from build123d import *

# Parameters (mm, degrees)
SKETCH1_R           = 11
BOSS_EXTRUDE1_DEPTH = 17.9
BOSS_EXTRUDE2_START = 32.2
SKETCH2_R           = 11
BOSS_EXTRUDE2_DEPTH = 32.2
BOSS_EXTRUDE3_DEPTH = 2.5
BOSS_EXTRUDE4_DEPTH = 15.3


# Read off the part's stored shape, not the designer's step: AdvancedHole1
with BuildPart() as part:
    # Sketch1 → Boss-Extrude1 (new body)
    with BuildSketch(Plane(origin=(0, 0, 0), x_dir=(0, 0, -1), z_dir=(1, 0, 0))):
        with Locations(Location((0, 0, 0), (0, 0, 180))):
            Circle(SKETCH1_R)
    extrude(amount=BOSS_EXTRUDE1_DEPTH)

    # Sketch2 → Boss-Extrude2 (add)
    with BuildSketch(Plane.ZY.offset(BOSS_EXTRUDE2_START)):
        Circle(SKETCH2_R)
    extrude(amount=-BOSS_EXTRUDE2_DEPTH)

    # Sketch3 → Cut-Revolve1 (revolve, cut)
    with BuildSketch(Plane.XY, mode=Mode.PRIVATE) as cut_revolve1_sk:
        with BuildLine():
            Line((0, 11), (0, 10))
            ThreePointArc((0, 10), (-0.292893219, 10.707106781), (-1, 11))
            Line((-1, 11), (0, 11))
        make_face()
    revolve(cut_revolve1_sk.sketch.rotate(Axis((17.9, 0, 0), (-1, 0, 0)), 270), axis=Axis((17.9, 0, 0), (-1, 0, 0)), mode=Mode.SUBTRACT)

    # Sketch4 → Boss-Extrude3 (add)
    with BuildSketch(Plane(origin=(17.9, 0, 0), x_dir=(0, 0, -1), z_dir=(1, 0, 0))):
        with BuildLine():
            ThreePointArc((4, 3), (2.236067977, 4.472135955), (0, 5))
            Line((0, 5), (0, -5))
            ThreePointArc((0, -5), (2.236067977, -4.472135955), (4, -3))
            Line((4, -3), (4, 3))
        make_face()
        with BuildLine():
            ThreePointArc((0, 5), (-2.236067977, 4.472135955), (-4, 3))
            Line((-4, 3), (-4, -3))
            ThreePointArc((-4, -3), (-2.236067977, -4.472135955), (0, -5))
            Line((0, -5), (0, 5))
        make_face()
    extrude(amount=BOSS_EXTRUDE3_DEPTH)

    # Sketch5 → Boss-Extrude4 (add)
    with BuildSketch(Plane(origin=(20.4, 0, 0), x_dir=(0, 0, -1), z_dir=(1, 0, 0))):
        with BuildLine():
            Line((0.968245837, 1.75), (-0.968245837, 1.75))
            ThreePointArc((-0.968245837, 1.75), (-1.015753003, -1.722859784), (2, 0))
            ThreePointArc((2, 0), (1.722859784, 1.015753003), (0.968245837, 1.75))
        make_face()
    extrude(amount=BOSS_EXTRUDE4_DEPTH)

    # AdvancedHole1 outline → AdvancedHole1 (revolve, cut)
    with BuildSketch(Plane(origin=(0, -9, 0), x_dir=(0, 1, 0), z_dir=(0, 0, -1))):
        Polygon((0, 14.219311505), (0.8, 14.7), (0.8, 17.9), (0, 17.9), align=None)
    revolve(axis=Axis((0, -9, 0), (1, 0, 0)), mode=Mode.SUBTRACT)

    # AdvancedHole1 2 outline → AdvancedHole1 2 (revolve, cut)
    with BuildSketch(Plane.YX.offset(9)):
        Polygon((0, 14.219311505), (0.8, 14.7), (0.8, 17.9), (0, 17.9), align=None)
    revolve(axis=Axis((0, 0, -9), (1, 0, 0)), mode=Mode.SUBTRACT)

    # AdvancedHole1 3 outline → AdvancedHole1 3 (revolve, cut)
    with BuildSketch(Plane.YX.offset(-9)):
        Polygon((0, 14.219311505), (0.8, 14.7), (0.8, 17.9), (0, 17.9), align=None)
    revolve(axis=Axis((0, 0, 9), (1, 0, 0)), mode=Mode.SUBTRACT)

    # AdvancedHole1 4 outline → AdvancedHole1 4 (revolve, cut)
    with BuildSketch(Plane(origin=(0, 9, 0), x_dir=(0, 1, 0), z_dir=(0, 0, -1))):
        Polygon((0, 14.219311505), (0.8, 14.7), (0.8, 17.9), (0, 17.9), align=None)
    revolve(axis=Axis((0, 9, 0), (1, 0, 0)), mode=Mode.SUBTRACT)


solid = part.part
Input: part model. Units: mm. Frame: model coordinates. A direction names the side the tool comes from. Coordinates: 2 decimals unless noted, no trailing zeros. Loops run counter-clockwise (first coordinate to the right, second up) from the corner with the lowest first, then second, coordinate; pieces in that order, holes last.
(1) Set-up query: faces 5 (the face through (28, 1.75, 0)), 6 (the face through (8.82, -10.74, -2.38)), 7 (the face through (19, 0, -4)), 8 (the face through (20.4, -1, -2)), 9 (the face through (19, 0, 4)). Return all of +Z, -Z, +X, -X, +Y, -Y with unobstructed straight access to the full face (end or side cutting, diameter ignored); none if empty.
(2) Pull-direction query (Z, two-part tool) for faces 1 (the face through (-16.82, -10.74, -2.38)), 2 (the face through (16.322, -0.104, 9.793)), 3 (the face through (-32.2, 0, 0)), 4 (the face through (14.303, -0.018, 9.138)); classes: released by +Z, released by -Z, zero draft, split by the parting line, or undercut.
(3) Section A-A on x = -13.5. Return the cut outline in (y, z), then the cut area to 3 significant figures.
(4) Material intervals for probe 1 along Z at (x, y) = (17.05, 0); probe 2 along X at (y, z) = (-6.5, -6); probe 3 along Z at (x, y) = (16.55, -9), sorted ascending.
(5) First-contact query: pin 1 Ø3 at (x, y) = (20, -5.5) entering from +Z; pin 2 Ø2.5 at (y, z) = (0, 9) entering from +X; pin 3 Ø0.6 at (x, z) = (30.5, 0.5) entering from +Y. Flat tips, straight axial feed; report the tip coordinate or a pass-through.
Data:
1. face 5: +Z, -Z, +X, +Y
1. face 6: +X, -X
1. face 7: -Z, +X, +Y, -Y
1. face 8: +X
1. face 9: +Z, +X, +Y, -Y
2. face 1: split by the parting line
2. face 2: undercut
2. face 3: zero draft
2. face 4: undercut
3. outline: circle Ø22 at (0, 0)
3. area: 380 mm2
4. probe 1: z = -11 to -9.8, -8.2 to 8.2, 9.8 to 11
4. probe 2: x = -32.2 to 17.9
4. probe 3: z = -6.32 to -0.8, 0.8 to 6.32
5. pin 1: stops at z = 3
5. pin 2: stops at x = 17.9
5. pin 3: stops at y = 1.75
